Source: three-view drawing plus pictorial views. Frame: mm from the lowest corner of the part. Give positions to 0.01 mm unless a question says otherwise; leave off trailing zeros. Loops run counter-clockwise (first coordinate to the right, second up) from the corner with the lowest first, then second, coordinate; pieces in that order, holes last. Notation, with made-up numbers: (29, 54.5) - (41, 54.5) arc R8 cw to (41, 66.5) - close; hole circle Ø11 at (-17.75, 74.5). An arc over 180 degrees is marked (long way). One line per item, written item: value.
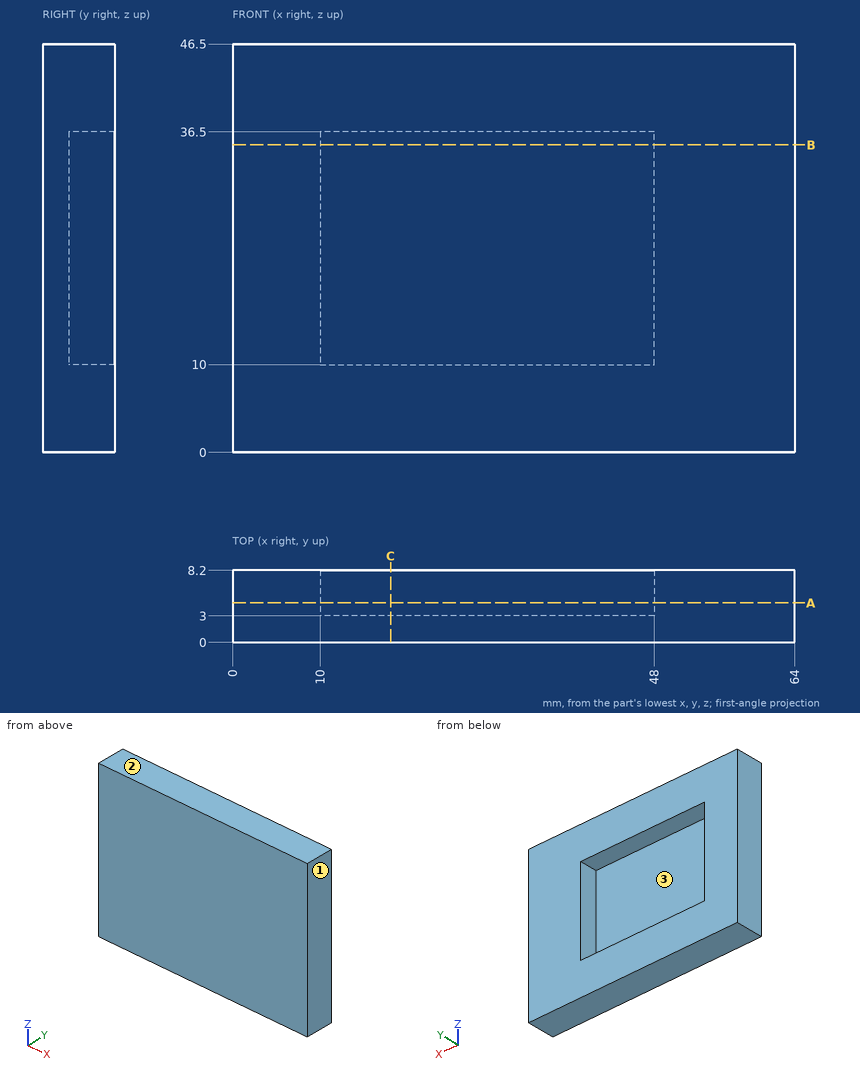
Item 1: Pin query (flat end, axial travel): P1, Ø10, axis at x = 14, z = 9, coming from the -Y side. Return the tip coordinate at first contact, or that it passes through.
Verdict:
P1: stops at y = 0
Item 2: Draft query along X for the marked faces 1, 2 and 3. Return one class per face: pulls with the +X half, pulls with the -X half, needs draft (parallel to the pull), parting line crosses it, or undercut.
Verdict:
face 1: pulls with the +X half
face 2: needs draft
face 3: undercut
Item 3: Section B-B, the plane z = 35. Output: boundary loops of the cut face in (x, y).
Verdict:
outline: (0, 0) - (64, 0) - (64, 8.2) - (48, 8.2) - (48, 3) - (10, 3) - (10, 8.2) - (0, 8.2) - close
Item 4: Section A-A, the plane y = 4.5. Output: boundary loops of the cut face in (x, z).
Verdict:
outline: (0, 0) - (64, 0) - (64, 46.5) - (0, 46.5) - close; hole (10, 10) - (48, 10) - (48, 36.5) - (10, 36.5) - close
Item 5: Section C-C, the plane x = 18. Output: boundary loops of the cut face in (y, z).
Verdict:
outline: (0, 0) - (8.2, 0) - (8.2, 10) - (3, 10) - (3, 36.5) - (8.2, 36.5) - (8.2, 46.5) - (0, 46.5) - close
Item 6: Material intervals for L1, parallel to X at y = 5.25, z = 13; L2, parallel to Z at x = 14, y = 5; L3, parallel to Y at x = 30.5, z = 16, sorted ascending.
Verdict:
L1: x = 0 to 10, 48 to 64
L2: z = 0 to 10, 36.5 to 46.5
L3: y = 0 to 3
